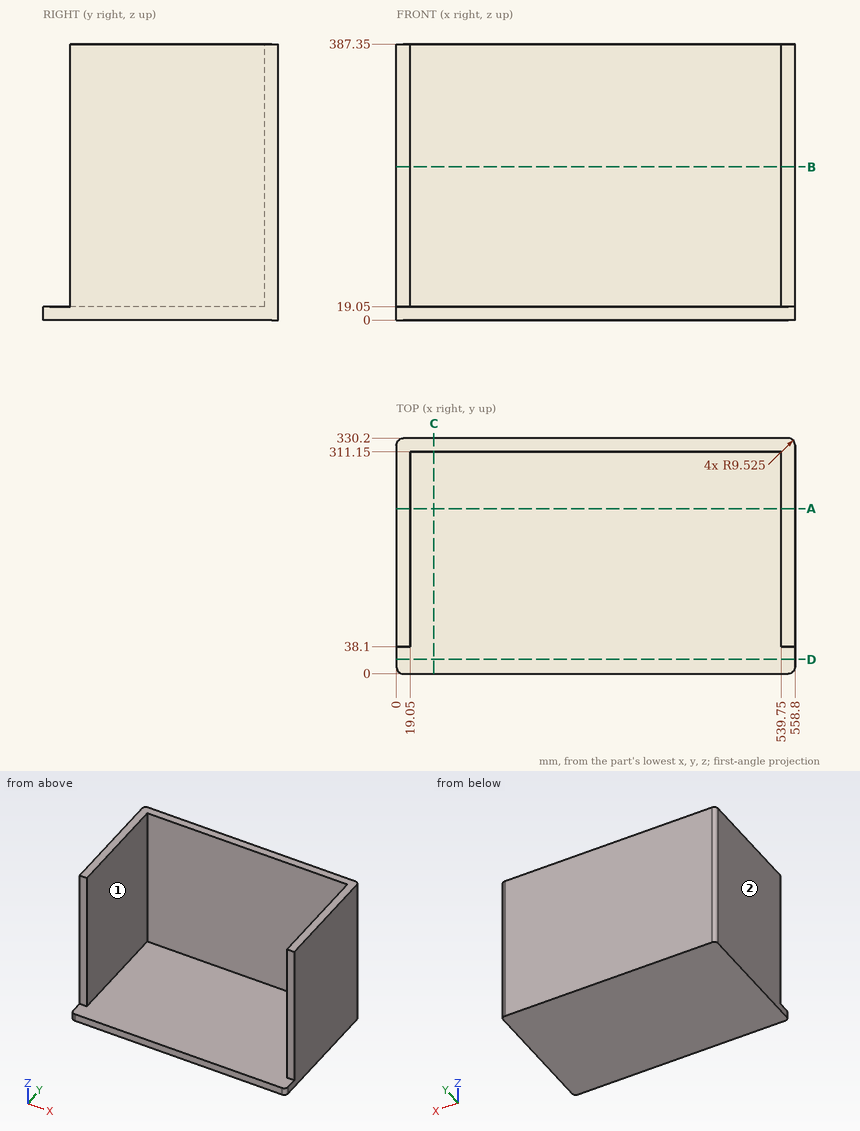
Can you work these out from the drawing? Everything is in mm from the part's minimum corner. A direction names the side the tool comes from. Round coordinates to 2 decimals unless told otherwise and drop trailing zeros. Loops run counter-clockwise (first coordinate to the right, second up) from the corner with the lowest first, then second, coordinate; pieces in that order, holes last. Notation, with made-up numbers: (71, -33) - (114, -33) arc R6 ccw to (114, -23) - close; hole circle Ø11 at (32, 83.25). An arc over 180 degrees is marked (long way). Write item = value, one per line. Start each with the question number.
(1) If we section it at B-B (z = 215): Please give me the cut outline in (x, y) (3 decimals).
(2) For P1, Ø21, axis at x = 546.5, z = 269, coming from the -Y side; P2, Ø10, axis at x = 460, z = 244.5, coming from the -Y side; P3, Ø8, axis at x = 219, y = 194, coming from the +Z side, each with a flat end and sliding along its axis, tell me the tip position at first contact or that it passes through.
(3) For the marked faces 1 and 2, which set-ups out of +Z, -Z, +X, -X, +Y, -Y let a thin tool reach every point of the face, with its end or its side?
(4) If we section it at A-A (y = 231.5): Please give me the cut outline in (x, z), and give its area (3 significant figures).
(5) If we section it at C-C (x = 52.5): Please give me the cut outline in (y, z).
(6) If I drill on probe 1 along X at (y, z) = (158.5, 125); probe 2 along Y at (x, z) = (461.5, 170.5); probe 3 along Z at (x, y) = (390.5, 201), over which ranges is the centre line in solid material (lowest first)? Write a range as [from, to].
(7) If we section it at D-D (y = 20): Please give me the cut outline in (x, z), and give its area (3 significant figures).
Ans:
q1.outline = (0, 38.1) - (19.05, 38.1) - (19.05, 311.15) - (539.75, 311.15) - (539.75, 38.1) - (558.8, 38.1) - (558.8, 320.675) arc R9.525 ccw to (549.275, 330.2) - (9.525, 330.2) arc R9.525 ccw to (0, 320.675) - close
q2.P1 = 38.1
q2.P2 = 311.15
q2.P3 = 19.05
q3.face_1 = +Z, -Y
q3.face_2 = +Z, -Z, -X, +Y, -Y
q4.outline = (0, 0) - (558.8, 0) - (558.8, 387.35) - (539.75, 387.35) - (539.75, 19.05) - (19.05, 19.05) - (19.05, 387.35) - (0, 387.35) - close
q4.area = 24,700 mm²
q5.outline = (0, 0) - (330.2, 0) - (330.2, 387.35) - (311.15, 387.35) - (311.15, 19.05) - (0, 19.05) - close
q6.probe_1 = [0, 19.05], [539.75, 558.8]
q6.probe_2 = [311.15, 330.2]
q6.probe_3 = [0, 19.05]
q7.outline = (0, 0) - (558.8, 0) - (558.8, 19.05) - (0, 19.05) - close
q7.area = 10,600 mm²
